The listing builds one solid part. Answer for the finished solid, in the listing's coordinates (mm). Coordinates: 2 decimals unless noted, no trailing zeros. Write each loop counter-clockwise with the first axis right and the second up, starting at its lowest first coordinate (ties: lowest second). Pieces come first, ordered by that corner, then holes.
Autodesk Fusion 360 part; units mm, degrees
sketch "Sketch1" plane through (0, 0, 0) normal (0, 0, 1) x (1, 0, 0)
  circle A0 centre (0, 0) radius 164
  line L0 (0, 220) -> (0, -226.5969) construction
  line L1 (-260, 0) -> (224.3647, 0) construction
  circle A1 centre (0, 164) radius 12.5
  line L2 (37, 164) -> (37, 118.79)
  line L3 (-37, 118.79) -> (-37, 164)
  arc A2 (37, 164) -> (-37, 164) centre (0, 164) ccw
  arc A3 (-164, 37) -> (-164, -37) centre (-164, 0) ccw
  circle A4 centre (-164, 0) radius 12.5
  line L4 (-118.79, -37) -> (-164, -37)
  line L5 (-164, 37) -> (-118.79, 37)
  arc A5 (-37, -164) -> (37, -164) centre (0, -164) ccw
  circle A6 centre (0, -164) radius 12.5
  line L6 (37, -118.79) -> (37, -164)
  line L7 (-37, -164) -> (-37, -118.79)
  arc A7 (164, -37) -> (164, 37) centre (164, 0) ccw
  circle A8 centre (164, 0) radius 12.5
  line L8 (118.79, 37) -> (164, 37)
  line L9 (164, -37) -> (118.79, -37)
  arc A9 (37, 118.79) -> (118.79, 37) centre (118.79, 118.79) ccw
  arc A10 (118.79, -37) -> (37, -118.79) centre (118.79, -118.79) ccw
  arc A11 (-37, -118.79) -> (-118.79, -37) centre (-118.79, -118.79) ccw
  arc A12 (-118.79, 37) -> (-37, 118.79) centre (-118.79, 118.79) ccw
  circle A13 centre (100, 0) radius 12.5
  circle A14 centre (0, 100) radius 12.5
  circle A15 centre (-100, 0) radius 12.5
  circle A16 centre (0, -100) radius 12.5
  circle A17 centre (0, 0) radius 49
  dimension "d1" = 328
  dimension "d3" = 74
  dimension "d4" = 25
  dimension "d7" = 45.21
  dimension "d8" = 45.21
  dimension "d10" = 360
  dimension "d11" = 25
  dimension "d12" = 100
  dimension "d14" = 360
  dimension "d15" = 98
extrude "Extrude1" add sketch "Sketch1" along normal blind 18 contours A0 A1 L2 L3 A4 L4 L5 A6 L6 L7 A8 L8 L9 A9 A10 A11 A12 | A0 A7 A8 L8 L9 | A0 A1 L2 L3 A2 | A0 A5 A6 L6 L7 | A0 A3 A4 L4 L5
fillet "Fillet2" radius 10 4 edges at (-111.6541, 4.5202, 0) (-11.6541, -95.4798, 0) (88.3459, 4.5202, 0) (-11.6541, 104.5202, 0)
scale "Scale1" factor 0.5 about (-164, 37, 18) bodies 1
equation "d3 = ( 37 * 2 ) * 1 mm"
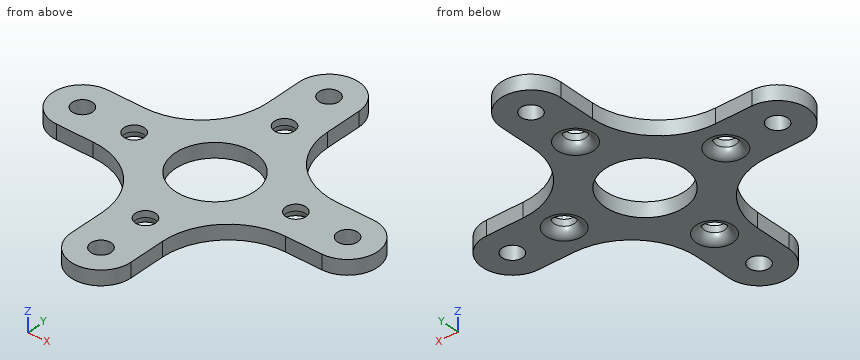
1. Find the intervals of material crossed by L1, parallel to Y at x = -84, z = 12.75; L2, parallel to X at y = 20, z = 12.5; L3, parallel to X at y = 30.5, z = 13.5, in increasing order.
Results found:
L1: y = -81.89 to -69.42, -57.58 to -37.59, -25.41 to -5.92, 42.92 to 62.41, 74.59 to 94.58, 106.42 to 118.89
L2: x = -182.44 to -170.07, -157.93 to -138.3, -125.7 to -106.45, -57.55 to -38.3, -25.7 to -6.07, 6.07 to 18.44
L3: x = -178.08 to -103.36, -60.64 to 14.08
2. Section A-A on z = 16 is taken. State how many separate pieces and enclosed holes the cut face has, then the cut area to 3 significant figures.
Results found:
separate pieces: 1
enclosed holes: 9
area: 11,500 mm2
3. Section D-D on x = -47 is taken. Give the vertices of the cut face in (y, z), then the cut area to 3 significant figures.
Results found:
outline: (-8.07, 9) - (45.07, 9) - (45.07, 18) - (-8.07, 18) - close
area: 478 mm2
4. Section B-B on y = 4.5 is taken. Give the vertices of the cut face in (x, z).
Results found:
outline: (-176.09, 9) - (-102.11, 9) - (-102.11, 18) - (-176.09, 18) - close; (-61.89, 9) - (12.09, 9) - (12.09, 18) - (-61.89, 18) - close
5. Section C-C on y = -31.5 is taken. Give the vertices of the cut face in (x, z).
Results found:
outline: (-101.59, 9) - (-93.25, 9) arc R5 ccw to (-88.25, 14) - (-88.25, 18) - (-101.59, 18) - close; (-75.75, 14) arc R5 ccw to (-70.75, 9) - (-62.41, 9) - (-62.41, 18) - (-75.75, 18) - close
6. Flat-ended cylindrical pins translate along their axes: P1, Ø2.5, axis at x = -156.5, z = 12.5, coming from the -Y side; P2, Ø1.5, axis at x = -26.5, z = 16.5, coming from the +Y side; P3, Ø5, axis at y = 86, z = 12, coming from the -X side. Find the tip coordinate at first contact, or state that the pin passes through.
Results found:
P1: stops at y = 0
P2: stops at y = 37.26
P3: stops at x = -100.5
